Geometry: see drawing. Coordinates: mm, zero at the bounding-box minimum. A direction names the side the tool comes from. Coordinates: 2 decimals unless noted, no trailing zeros. Write each loop counter-clockwise with the first axis right and the second up, starting at its lowest first coordinate (ties: lowest second). Pieces come first, ordered by that corner, then holes. Notation, with made-up numbers: M -37,48 L -20,48 A24 ccw -20,58 Z; hole C 23,-33 d9. An arc over 180 degrees is marked long. One line per item, written item: value. Start each with the question number.
Item 1: Pin query (flat end, axial travel): P1, Ø10, axis at x = 53, z = 17, coming from the +Y side; P2, Ø3, axis at y = 29.5, z = 24, coming from the +X side; P3, Ø1, axis at x = 41, z = 14, coming from the -Y side; P4, Ø8, axis at x = 7.5, y = 10, coming from the -Z side. Return the tip coordinate at first contact, or that it passes through.
Item 2: Set-up query: the marked faces 1, 2 and 3. Return all of +Z, -Z, +X, -X, +Y, -Y with unobstructed straight access to the full face (end or side cutting, diameter ignored); none if empty.
Item 3: Cut plane D-D, the plane x = 63. Output: boundary loops of the cut face in (y, z), then the cut area to 3 significant figures.
Item 4: Cut plane B-B, the plane y = 31.5. Output: boundary loops of the cut face in (x, z), then the cut area to 3 significant figures.
Item 5: Cut plane C-C, the plane x = 10. Output: boundary loops of the cut face in (y, z), then the cut area to 3 significant figures.
Item 6: Ray query, L1, parallel to Y at x = 25, z = 18; L2, parallel to Z at x = 25.4, y = 10.8; L3, parallel to X at y = 7.5, z = 4.5. Return the intervals inside material, ascending. Write a range as from..to.
Item 7: Cut plane A-A, the plane z = 34. Output: boundary loops of the cut face in (x, y), then the cut area to 3 significant figures.
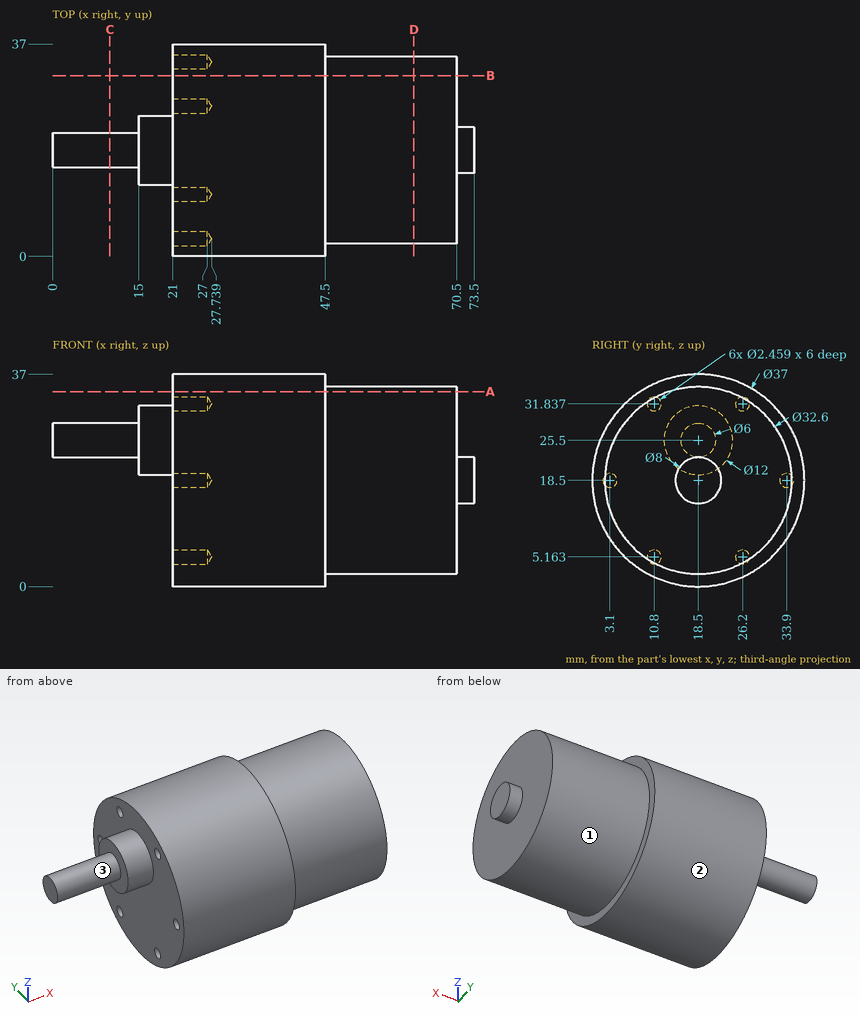
From the geometry:
1. P1: stops at y = 34.8
1. P2: stops at x = 70.5
1. P3: stops at y = 0.44
1. P4: passes through
2. face 1: +X
2. face 2: +X, -X
2. face 3: -X
3. outline: C 18.5,18.5 d32.6
3. area: 835 mm²
4. outline: M 21,5.34 L 47.5,5.34 L 47.5,8.67 L 70.5,8.67 L 70.5,28.33 L 47.5,28.33 L 47.5,31.66 L 21,31.66 Z
4. area: 1,150 mm²
5. outline: C 18.5,25.5 d6
5. area: 28.3 mm²
6. L1: y = 0.01..1.98, 4.22..32.78, 35.02..36.99
6. L2: z = 1.68..3.93, 6.39..30.61, 33.07..35.32
6. L3: x = 21..47.5
7. outline: M 21,8.4 L 47.5,8.4 L 47.5,13.46 L 70.5,13.46 L 70.5,23.54 L 47.5,23.54 L 47.5,28.6 L 21,28.6 Z
7. area: 767 mm²
